Can you work these out from the model? Positions are in its coordinate system, mm. Round coordinates to 2 decimals unless told otherwise and drop trailing zeros. Order: outer loops, then holes, each group sorted by start corner. A loop starts at its lowest first (then second) coordinate and runs counter-clockwise, first axis right, second up. Notation, with made-up numbers: M 56.5,70.25 L 78.5,70.25 A25 ccw 78.5,106.25 Z; hole C -33.75,19 d4. An arc over 180 degrees is marked long. One line per question, with ' | ' between items.
```python
from build123d import *

# Parameters (mm, degrees)
F0_W      = 50.4710152745
F0_H      = 52.5459498167
F1_DEPTH  = 128.1304806471
F2_T      = -2.54
F4_DEPTH  = 87.9370719194
F5_DEPTH  = 92.566229403
F6_DEPTH  = 25.4
F7_DEPTH  = 25.4
F8_DEPTH  = 25.4
F9_DEPTH  = 74.4861587882
F10_W     = 31.4560076222
F10_H     = 22.1310183406
F11_DEPTH = 25.4
F12_R     = 11.5820249722
F13_DEPTH = 25.4


with BuildPart() as f1:
    # F0 (on Top) → F1 (new body)
    with BuildSketch(Plane.XY):
        Rectangle(F0_W, F0_H)
    extrude(amount=F1_DEPTH)

    # F2
    f2_openings = [f1.faces().sort_by_distance(p)[0] for p in [
        (0, 0, 128.130481),
    ]]
    offset(amount=F2_T, openings=f2_openings)

    # F3 (on face) → F4 (cut)
    with BuildSketch(Plane.XZ.offset(26.2729749084)):
        with BuildLine():
            add(Edge.make_bspline(
                [(0, 13.7362796813), (7.3372486719, 13.7362796813), (3.6686243359, 97.3400166258), (0, 180.9437535703), (-3.6686243359, 97.3400166258), (-7.3372486719, 13.7362796813), (0, 13.7362796813)],
                knots=[0, 0, 0, 2.0943951024, 2.0943951024, 4.1887902048, 4.1887902048, 6.2831853072, 6.2831853072, 6.2831853072], degree=2, weights=[1, 0.5, 1, 0.5, 1, 0.5, 1]))
        make_face()
    extrude(amount=-F4_DEPTH, mode=Mode.SUBTRACT)

    # F5 (cut): a face of the model
    f5_faces = [f1.faces().sort_by_distance(p)[0] for p in [
        (0, 23.7329749084, 126.7950663606),
    ]]
    extrude(f5_faces, amount=F5_DEPTH, mode=Mode.SUBTRACT)

    # F6 (cut): a face of the model
    f6_faces = [f1.faces().sort_by_distance(p)[0] for p in [
        (0, 23.7329749084, 126.7950663606),
    ]]
    extrude(f6_faces, amount=-F6_DEPTH, mode=Mode.SUBTRACT)

    # F7 (cut): a face of the model
    f7_faces = [f1.faces().sort_by_distance(p)[0] for p in [
        (0, 0, 2.54),
    ]]
    extrude(f7_faces, amount=-F7_DEPTH, mode=Mode.SUBTRACT)

    # F8 (cut): a face of the model
    f8_faces = [f1.faces().sort_by_distance(p)[0] for p in [
        (-22.6955076373, 0, 64.0652403235),
    ]]
    extrude(f8_faces, amount=-F8_DEPTH, mode=Mode.SUBTRACT)

    # F9 (add): a face of the model
    f9_faces = [f1.faces().sort_by_distance(p)[0] for p in [
        (23.9655076373, 0, 128.1304806471),
    ]]
    extrude(f9_faces, amount=F9_DEPTH)

    # F10 (on face) → F11 (cut)
    with BuildSketch(Plane(origin=(22.6955076373, 0, 0), x_dir=(0, -1, 0), z_dir=(-1, 0, 0))):
        with Locations((-0.7681553252, 191.551130265)):
            Rectangle(F10_W, F10_H)
    extrude(amount=-F11_DEPTH, mode=Mode.SUBTRACT)

    # F12 (on face) → F13 (cut)
    with BuildSketch(Plane(origin=(22.6955076373, 0, 0), x_dir=(0, -1, 0), z_dir=(-1, 0, 0))):
        with Locations((0, 16.72661677)):
            Circle(F12_R)
    extrude(amount=-F13_DEPTH, mode=Mode.SUBTRACT)


solid = f1.part
```
(1) Thinking about a two-plate mould opening in Y: for faces 1 (the flat face through (25.236, 0, 100)), 2 (the cylindrical face through (23.95, 1.51, 28.21)), which applies, released by +Y, released by -Y, zero draft, split by the parting line, or undercut?
Final values:
face 1: zero draft | face 2: undercut
(2) If we section it at B-B on x = 24.8: Please give me the cut outline in (y, z).
Final values:
outline: M -26.27,0 L 26.27,0 L 26.27,202.62 L 16.5,202.62 L 16.5,180.49 L -14.96,180.49 L -14.96,202.62 L -26.27,202.62 Z; hole C 0,16.73 d23.16
(3) Will this pin go through, and if not, where does the flat tip stop? pin 1 Ø1.3 at (x, y) = (23.5, -1) entering from +Z.
Final values:
pin 1: z = 180.49
(4) Please list where these lines run through material, in increasing order: probe 1 along Z at (x, y) = (23.85, 0); probe 2 along Z at (x, y) = (24.05, 12); probe 3 along Z at (x, y) = (25.1, -4.5). Write a range as [from, to].
Final values:
probe 1: [0, 5.14], [28.31, 180.49] | probe 2: [0, 180.49] | probe 3: [0, 6.05], [27.4, 180.49]
(5) If we section it at A-A on y = 0: Please give me the cut outline in (x, z), plus the area to 3 significant figures.
Final values:
outline: M 22.7,0 L 25.24,0 L 25.24,5.14 L 22.7,5.14 Z; M 22.7,28.31 L 25.24,28.31 L 25.24,180.49 L 22.7,180.49 Z | area: 400 mm^2
